Source: CAD feature listing. Evaluate the final solid. Frame: model axes, mm. A direction names the side the tool comes from. Give positions to 0.01 mm unless a question says otherwise; leave off trailing zeros. Write each loop counter-clockwise with the first axis right and the second up, starting at its lowest first coordinate (ties: lowest second). Pieces come first, ordered by that corner, then holes.
```python
from build123d import *

# Parameters (mm, degrees)
SKETCH1_W           = 6.35
SKETCH1_H           = 6.35
SKETCH1_R           = 3.6703
BOSS_EXTRUDE1_DEPTH = 6.35
SKETCH2_R           = 1.5
CUT_EXTRUDE1_DEPTH  = 7.35


with BuildPart() as part:
    # Sketch1 → Boss-Extrude1 (new body)
    with BuildSketch(Plane(origin=(0, 0, 0), x_dir=(1, 0, 0), z_dir=(0, 1, 0))):
        Polygon((0, 25.4), (0, 0), (20.0406, 0), (20.0406, 25.4), (13.6906, 25.4), (13.6906, 44.45), (20.0406, 44.45), (20.0406, 69.85), (0, 69.85), (0, 44.45), (6.35, 44.45), (6.35, 25.4), align=None)
        with Locations((10.0203, 6.35)):
            Rectangle(SKETCH1_W, SKETCH1_H, mode=Mode.SUBTRACT)
        with Locations((10.0203, 22.225)):
            Circle(SKETCH1_R, mode=Mode.SUBTRACT)
        with Locations((10.0203, 63.5)):
            Rectangle(SKETCH1_W, SKETCH1_H, mode=Mode.SUBTRACT)
        with Locations((10.0203, 47.625)):
            Circle(SKETCH1_R, mode=Mode.SUBTRACT)
    extrude(amount=BOSS_EXTRUDE1_DEPTH)

    # Sketch2 → Cut-Extrude1 (cut, through all)
    with BuildSketch(Plane(origin=(0, 6.35, 0), x_dir=(1, 0, 0), z_dir=(0, 1, 0))):
        with Locations((3.175, 50.8)):
            Circle(SKETCH2_R)
        with Locations((3.175, 19.05)):
            Circle(SKETCH2_R)
        with Locations((16.8656, 19.05)):
            Circle(SKETCH2_R)
        with Locations((16.8656, 50.8)):
            Circle(SKETCH2_R)
    extrude(amount=-CUT_EXTRUDE1_DEPTH, mode=Mode.SUBTRACT)


solid = part.part
```
1. Section query A-A (x = 10.25). Return loops of the section in (y, z) (3 decimals), plus the area to 3 significant figures.
2. Pull-direction query (X, two-part tool) for faces 4 (the flat face through (10, 3, -9.525)), 5 (the flat face through (0, 3, -13)), 6 (the flat face through (17, 3, -44.45)), 7 (the flat face through (20.041, 3, -57)); classes: pulls with the +X half, pulls with the -X half, needs draft (parallel to the pull), parting line crosses it, or undercut.
3. Access query for faces 1 (the flat face through (10, 0, -35)), 2 (the flat face through (6.35, 3, -35)), 3 (the flat face through (10, 3, -66.675)). Directions: +Z, -Z, +X, -X, +Y, -Y. A direction counts if a zero-diameter tool reaches every point of the face in a straight line with its end or side. Return the directions, or none.
4. Section query D-D (x = 16.75). Return loops of the section in (y, z).
5. Line query: probe 1 along Z at (x, y) = (10, 6.25) (3 decimals); probe 2 along Z at (x, y) = (3.25, 3); probe 3 along Z at (x, y) = (7.5, 5.5) (3 decimals). Output: solid intervals per line, ascending.
6. Section query C-C (y = 2). Give the number of separate pieces and of enclosed holes in the cut face, plus the area to 3 significant figures.
7. Pin query (flat end, axial travel): P1, Ø3.5, axis at x = 3.175, z = -19.05, coming from the +Y side; P2, Ø3, axis at y = 3.5, z = -31, coming from the -X side. Return the tip coordinate at first contact, or that it passes through.
8. Section query B-B (z = -47). Return loops of the section in (x, y), plus the area to 3 significant figures.
The answers:
1. outline: (0, -69.85) - (6.35, -69.85) - (6.35, -66.675) - (0, -66.675) - close; (0, -60.325) - (6.35, -60.325) - (6.35, -51.288) - (0, -51.288) - close; (0, -43.962) - (6.35, -43.962) - (6.35, -25.888) - (0, -25.888) - close; (0, -18.562) - (6.35, -18.562) - (6.35, -9.525) - (0, -9.525) - close; (0, -3.175) - (6.35, -3.175) - (6.35, 0) - (0, 0) - close
1. area: 270 mm2
2. face 4: undercut
2. face 5: pulls with the -X half
2. face 6: needs draft
2. face 7: pulls with the +X half
3. face 1: +Z, -Z, +X, -X, -Y
3. face 2: -X, +Y, -Y
3. face 3: +Y, -Y
4. outline: (0, -69.85) - (6.35, -69.85) - (6.35, -52.3) - (0, -52.3) - close; (0, -49.3) - (6.35, -49.3) - (6.35, -44.45) - (0, -44.45) - close; (0, -25.4) - (6.35, -25.4) - (6.35, -20.55) - (0, -20.55) - close; (0, -17.55) - (6.35, -17.55) - (6.35, 0) - (0, 0) - close
5. probe 1: z = -69.85 to -66.675, -60.325 to -51.295, -43.955 to -25.895, -18.555 to -9.525, -3.175 to 0
5. probe 2: z = -69.85 to -52.3, -49.3 to -44.45, -25.4 to -20.55, -17.55 to 0
5. probe 3: z = -69.85 to -66.675, -60.325 to -50.293, -44.957 to -24.893, -19.557 to -9.525, -3.175 to 0
6. separate pieces: 1
6. enclosed holes: 8
6. area: 964 mm2
7. P1: stops at y = 6.35
7. P2: stops at x = 6.35
8. outline: (0, 0) - (6.4, 0) - (6.4, 6.35) - (0, 6.35) - close; (13.64, 0) - (20.04, 0) - (20.04, 6.35) - (13.64, 6.35) - close
8. area: 81.3 mm2
